The listing builds one solid part. Answer for the finished solid, in the listing's coordinates (mm). A direction names the side the tool comes from. Give positions to 0.01 mm unless a question says otherwise; leave off trailing zeros. Write each loop counter-clockwise with the first axis right and the second up, starting at its lowest first coordinate (ties: lowest second). Pieces come first, ordered by that corner, then holes. Notation, with made-up numbers: (82.5, -5.5) - (103.5, -5.5) arc R3 ccw to (103.5, -1.5) - close; hole circle Ø1 at (24, 10.25). An arc over 180 degrees is marked (long way). One line per item, written item: value. Start each with the question number.
from build123d import *

# Parameters (mm, degrees)
F1_DEPTH = 76
F2_W     = 1
F2_H     = 3.5
F2_W_2   = 19
F3_DEPTH = 50.001
F5_DEPTH = 48.5


# Not quite as in the source:
# - a feature names something its author has since deleted; it is built from what else it names


with BuildPart() as f1:
    # F0 (on Top) → F1 (new body)
    with BuildSketch(Plane.XY):
        with BuildLine():
            ThreePointArc((-1, 0), (-0.2928932188, 0.2928932188), (0, 1))
            Line((0, 1), (0, 47))
            ThreePointArc((0, 47), (0.2928932188, 47.7071067812), (1, 48))
            Line((1, 48), (55, 48))
            ThreePointArc((55, 48), (55.7071067812, 47.7071067812), (56, 47))
            Line((56, 47), (56, 1))
            ThreePointArc((56, 1), (56.2928932188, 0.2928932188), (57, 0))
            Line((57, 0), (64, 0))
            ThreePointArc((64, 0), (64.7071067812, 0.2928932188), (65, 1))
            ThreePointArc((65, 1), (64.7071067812, 1.7071067812), (64, 2))
            Line((64, 2), (59, 2))
            ThreePointArc((59, 2), (58.2928932188, 2.2928932188), (58, 3))
            Line((58, 3), (58, 49))
            ThreePointArc((58, 49), (57.7071067812, 49.7071067812), (57, 50))
            Line((57, 50), (-1, 50))
            ThreePointArc((-1, 50), (-1.7071067812, 49.7071067812), (-2, 49))
            Line((-2, 49), (-2, 1))
            ThreePointArc((-2, 1), (-1.7071067812, 0.2928932188), (-1, 0))
        make_face()
    extrude(amount=F1_DEPTH)

    # F2 (on face) → F3 (cut, through all)
    with BuildSketch(Plane(origin=(0, 50, 0), x_dir=(-1, 0, 0), z_dir=(0, 1, 0))):
        with Locations((1.5, 17.75)):
            Rectangle(F2_W, F2_H)
        with Locations((-8.5, 17.75)):
            Rectangle(F2_W_2, F2_H)
        with Locations((-8.5, 40.25)):
            Rectangle(F2_W_2, F2_H)
        with Locations((-8.5, 62.75)):
            Rectangle(F2_W_2, F2_H)
        with Locations((1.5, 40.25)):
            Rectangle(F2_W, F2_H)
        with Locations((1.5, 62.75)):
            Rectangle(F2_W, F2_H)
    extrude(amount=-F3_DEPTH, mode=Mode.SUBTRACT)

    # F4 (on face) → F5 (join, through all)
    with BuildSketch(Plane.XY.offset(16)):
        with BuildLine():
            ThreePointArc((0, 47), (-1, 48), (-2, 47))
            ThreePointArc((-2, 47), (-1, 46), (0, 47))
        make_face()
        with BuildLine():
            ThreePointArc((0, 24), (-1, 25), (-2, 24))
            ThreePointArc((-2, 24), (-1, 23), (0, 24))
        make_face()
        with BuildLine():
            ThreePointArc((0, 1), (-1, 2), (-2, 1))
            ThreePointArc((-2, 1), (-1, 0), (0, 1))
        make_face()
        with BuildLine():
            ThreePointArc((0.999999997, 50), (0, 48.9999999985), (1, 48))
            ThreePointArc((1, 48), (1.7071067812, 48.2928932188), (2, 49))
            ThreePointArc((2, 49), (1.7071067801, 49.7071067822), (0.999999997, 50))
        make_face()
    extrude(amount=F5_DEPTH)


solid = f1.part
Item 1: Find section B-B on x = 7. Determine the outline of the cut face in (y, z).
Item 2: Each of these flat-tipped pins is pushed along its axis until it touches: pin 1 Ø4 at (x, z) = (49, 29) entering from -Y; pin 2 Ø21 at (y, z) = (13.5, 55) entering from +X; pin 3 Ø2.5 at (x, z) = (60.5, 26) entering from +Y. Where does it stop, or does it pass through?
Item 3: Find section A-A on y = 13. Determine the outline of the cut face in (x, z), plus the area to 3 significant figures.
Item 4: The mould has two halves that part along Z. Classify faces 5 (the flat face through (-1, 36, 16)), 6 (the flat face through (58, 26, 37)), 7 (the flat face through (29, 49, 76)): +Z half, -Z half, draft (parallel to the pull), parting line (faces both ways), or undercut.
Item 5: For faces 1 (the flat face through (0, 24, 70)), 2 (the flat face through (18, 49, 40)), 3 (the flat face through (28, 50, 37)), 4 (the cylindrical face through (-1, 46, 18)), determine the directions among +Z, -Z, +X, -X, +Y, -Y from which every point of the face is accessible in a straight line to the end or side of a thin tool.
Item 6: Straight lines are drawn through the part: line 1 along X through (y, z) = (3, 29); line 2 along X through (y, z) = (39, 64); line 3 along Y through (x, z) = (59, 47.5). For each, find the intervals that lie inside material, in ascending order.
Item 7: Find section D-D on x = 51. Determine the outline of the cut face in (y, z).
Item 8: Find section C-C on z = 56. Determine the outline of the cut face in (x, y).
Values:
1. outline: (48, 0) - (50, 0) - (50, 16) - (48, 16) - close; (48, 19.5) - (50, 19.5) - (50, 38.5) - (48, 38.5) - close; (48, 42) - (50, 42) - (50, 61) - (48, 61) - close; (48, 64.5) - (50, 64.5) - (50, 76) - (48, 76) - close
2. pin 1: y = 48
2. pin 2: x = 58
2. pin 3: y = 2
3. outline: (-2, 0) - (0, 0) - (0, 16) - (-2, 16) - close; (-2, 19.5) - (0, 19.5) - (0, 38.5) - (-2, 38.5) - close; (-2, 42) - (0, 42) - (0, 61) - (-2, 61) - close; (-2, 64.5) - (0, 64.5) - (0, 76) - (-2, 76) - close; (56, 0) - (58, 0) - (58, 76) - (56, 76) - close
3. area: 283 mm^2
4. face 5: undercut
4. face 6: draft
4. face 7: +Z half
5. face 1: +Z, -Z, -Y
5. face 2: +Y, -Y
5. face 3: +Z, -Z, +X, -X, +Y
5. face 4: none
6. line 1: -2 to 0, 56 to 58
6. line 2: 56 to 58
6. line 3: 0 to 2
7. outline: (48, 0) - (50, 0) - (50, 76) - (48, 76) - close
8. outline: (-2, 1) arc R1 ccw to (0, 1) - (0, 47) arc R1 cw to (1, 48) - (55, 48) arc R1 cw to (56, 47) - (56, 1) arc R1 ccw to (57, 0) - (64, 0) arc R1 ccw to (64, 2) - (59, 2) arc R1 cw to (58, 3) - (58, 49) arc R1 ccw to (57, 50) - (-1, 50) arc R1 ccw to (-2, 49) - close
